from build123d import *

# Parameters (mm, degrees)
SKETCH_1_R          = 5
EXTRUDE_4_DEPTH     = 10
SKETCH_4_R          = 4
EXTRUDE_5_DEPTH     = 10
EXTRUDE_START       = 10
SKETCH_5_R          = 4
EXTRUDE_6_DEPTH     = 10
EXTRUDE_START_2     = -3
SKETCH_6_W          = 4.7
SKETCH_6_H          = 4.7
EXTRUDE_7_DEPTH     = 3
CUT_EXTRUDE_START   = -5
CUT_EXTRUDE_1_DEPTH = 5
SKETCH_8_R          = 1.5
CUT_EXTRUDE_2_DEPTH = 32.98820095


with BuildPart() as part:
    # 草图1 → 凸台-拉伸4 (new body)
    with BuildSketch(Plane(origin=(0, 0, 0), x_dir=(1, 0, 0), z_dir=(0, 1, 0))):
        with Locations(Location((0, 0, 0), (0, 0, 270))):
            Circle(SKETCH_1_R)
    extrude(amount=EXTRUDE_4_DEPTH)

    # 草图4 → 凸台-拉伸5 (add)
    with BuildSketch(Plane(origin=(0, 10, 0), x_dir=(1, 0, 0), z_dir=(0, 1, 0))):
        with Locations(Location((0, 0, 0), (0, 0, 270))):
            Circle(SKETCH_4_R)
    extrude(amount=EXTRUDE_5_DEPTH)

    # 草图5 → 凸台-拉伸6 (add)
    with BuildSketch(Plane.XZ.offset(EXTRUDE_START)):
        with Locations(Location((0, 0, 0), (0, 0, 90))):
            Circle(SKETCH_5_R)
    extrude(amount=-EXTRUDE_6_DEPTH)

    # 草图6 → 凸台-拉伸7 (add)
    with BuildSketch(Plane(origin=(0, 20, 0), x_dir=(1, 0, 0), z_dir=(0, 1, 0)).offset(EXTRUDE_START_2)):
        with BuildLine():
            Line((-7.85, 2.35), (-7.85, -2.35))
            Line((-7.85, -2.35), (-3.236896662, -2.35))
            ThreePointArc((-3.236896662, -2.35), (-4, 0), (-3.236896662, 2.35))
            Line((-3.236896662, 2.35), (-7.85, 2.35))
        make_face()
        with BuildLine():
            Line((-2.35, 7.85), (-2.35, 3.236896662))
            ThreePointArc((-2.35, 3.236896662), (0, 4), (2.35, 3.236896662))
            Line((2.35, 3.236896662), (2.35, 7.85))
            Line((2.35, 7.85), (-2.35, 7.85))
        make_face()
        with BuildLine():
            ThreePointArc((4, 0), (3.804443892, -1.235397376), (3.236896662, -2.35))
            Line((3.236896662, -2.35), (7.85, -2.35))
            Line((7.85, -2.35), (7.85, 2.35))
            Line((7.85, 2.35), (3.236896662, 2.35))
            ThreePointArc((3.236896662, 2.35), (3.804443892, 1.235397376), (4, 0))
        make_face()
        with BuildLine():
            ThreePointArc((2.35, -3.236896662), (0, -4), (-2.35, -3.236896662))
            Line((-2.35, -3.236896662), (-2.35, -7.85))
            Line((-2.35, -7.85), (2.35, -7.85))
            Line((2.35, -7.85), (2.35, -3.236896662))
        make_face()
        with BuildLine():
            Line((2.35, -2.35), (-2.35, -2.35))
            Line((-2.35, -2.35), (-2.35, -3.236896662))
            ThreePointArc((-2.35, -3.236896662), (0, -4), (2.35, -3.236896662))
            Line((2.35, -3.236896662), (2.35, -2.35))
        make_face()
        with BuildLine():
            Line((2.35, 2.35), (2.35, -2.35))
            Line((2.35, -2.35), (3.236896662, -2.35))
            ThreePointArc((3.236896662, -2.35), (3.804443892, -1.235397376), (4, 0))
            ThreePointArc((4, 0), (3.804443892, 1.235397376), (3.236896662, 2.35))
            Line((3.236896662, 2.35), (2.35, 2.35))
        make_face()
        with BuildLine():
            Line((-2.35, 3.236896662), (-2.35, 2.35))
            Line((-2.35, 2.35), (2.35, 2.35))
            Line((2.35, 2.35), (2.35, 3.236896662))
            ThreePointArc((2.35, 3.236896662), (0, 4), (-2.35, 3.236896662))
        make_face()
        with BuildLine():
            ThreePointArc((-3.236896662, 2.35), (-4, 0), (-3.236896662, -2.35))
            Line((-3.236896662, -2.35), (-2.35, -2.35))
            Line((-2.35, -2.35), (-2.35, 2.35))
            Line((-2.35, 2.35), (-3.236896662, 2.35))
        make_face()
        Rectangle(SKETCH_6_W, SKETCH_6_H)
    extrude(amount=EXTRUDE_7_DEPTH)

    # 草图7 → 切除-拉伸1 (cut)
    with BuildSketch(Plane(origin=(0, 20, 0), x_dir=(1, 0, 0), z_dir=(0, 1, 0)).offset(CUT_EXTRUDE_START)):
        with BuildLine():
            Line((-2.35, -2.35), (-3.236896662, -2.35))
            ThreePointArc((-3.236896662, -2.35), (-2.828427125, -2.828427125), (-2.35, -3.236896662))
            Line((-2.35, -3.236896662), (-2.35, -2.35))
        make_face()
        with BuildLine():
            Line((3.236896662, -2.35), (2.35, -2.35))
            Line((2.35, -2.35), (2.35, -3.236896662))
            ThreePointArc((2.35, -3.236896662), (2.828427125, -2.828427125), (3.236896662, -2.35))
        make_face()
        with BuildLine():
            Line((2.35, 3.236896662), (2.35, 2.35))
            Line((2.35, 2.35), (3.236896662, 2.35))
            ThreePointArc((3.236896662, 2.35), (2.828427125, 2.828427125), (2.35, 3.236896662))
        make_face()
        with BuildLine():
            ThreePointArc((-2.35, 3.236896662), (-2.828427125, 2.828427125), (-3.236896662, 2.35))
            Line((-3.236896662, 2.35), (-2.35, 2.35))
            Line((-2.35, 2.35), (-2.35, 3.236896662))
        make_face()
    extrude(amount=CUT_EXTRUDE_1_DEPTH, mode=Mode.SUBTRACT)

    # 草图8 → 切除-拉伸2 (cut, through all)
    with BuildSketch(Plane(origin=(0, 20, 0), x_dir=(1, 0, 0), z_dir=(0, 1, 0))):
        with Locations(Location((0, 0, 0), (0, 0, 270))):
            Circle(SKETCH_8_R)
    extrude(amount=-CUT_EXTRUDE_2_DEPTH, mode=Mode.SUBTRACT)


solid = part.part
The model under review builds one solid part; all positions refer to its coordinate system, in mm. A direction names the side the tool comes from. Round coordinates to 2 decimals unless told otherwise and drop trailing zeros. Order: outer loops, then holes, each group sorted by start corner. A loop starts at its lowest first (then second) coordinate and runs counter-clockwise, first axis right, second up. Notation, with made-up numbers: (55, 9) -> (89, 9) arc R14 ccw to (89, 31) -> close; hole circle Ø1 at (-34, -19). An arc over 180 degrees is marked (long way). Use CSV: the item, a comma, the result in double quotes. Start each with the question number.
(1) Tool access review of faces 5 (the face through (4, 18, -2.35)), 6 (the face through (2.35, 18, 4)), 7 (the face through (-5, 19, 2.35)), 8 (the face through (-4, 18, -2.35)): name each direction out of +Z, -Z, +X, -X, +Y, -Y from which nothing blocks a thin tool from reaching the whole face with its end or side.
(2) Insertion check: pin 1 (4 mm diameter, centred on y = 17, z = 6, fed in from +X); pin 2 (1 mm diameter, centred on x = -4.5, y = 1.5, fed in from +Z); pin 3 (4 mm diameter, centred on x = -4.5, y = 16.5, fed in from -Z). Each pin has a flat end and moves straight along its axis. Give the tip position at first contact, or say it passes through.
(3) Wall thickness on probe 1 along X at (y, z) = (-1.25, 0); probe 2 along X at (y, z) = (0.5, 0); probe 3 along Y at (x, z) = (5.5, -2.25): over which ranges is each line inside the solid? List them lowest first. Write a range as from..to.
(4) Consider section B-B on z = 0. Write out the cut boundary in (x, y).
(5) Consider section C-C on y = 16.25. Write out the cut boundary in (x, z), and give its area (3 significant figures).
(6) Mouldability with a two-part tool opening along Y and no side actions: class faces 1 (the face through (0, 17, -6)), 2 (the face through (0, 18, -7.85)), 3 (the face through (-2.7, 15, -2.7)), 4 (the face through (0, 17, 6)) as pulls with the +Y half, pulls with the -Y half, needs draft (parallel to the pull), parting line crosses it, or undercut.
(7) Consider section D-D on z = -2.75. Write out the cut boundary in (x, y), and give its area (3 significant figures).
(8) Consider section A-A on x = 0. Write out the cut boundary in (y, z).
Responses:
1,face 5,"-Z, +X, +Y"
1,face 6,"+Z, +X, +Y"
1,face 7,"+Z, -X, +Y"
1,face 8,"-Z, -X, +Y"
2,pin 1,"x = 2.35"
2,pin 2,"z = 3"
2,pin 3,"z = -2.43"
3,probe 1,"-4..-1.5, 1.5..4"
3,probe 2,"-5..-1.5, 1.5..5"
3,probe 3,"17..20"
4,outline,"(-7.85, 17) -> (-4, 17) -> (-4, 10) -> (-5, 10) -> (-5, 0) -> (-4, 0) -> (-4, -10) -> (-1.5, -10) -> (-1.5, 20) -> (-7.85, 20) -> close; (1.5, -10) -> (4, -10) -> (4, 0) -> (5, 0) -> (5, 10) -> (4, 10) -> (4, 17) -> (7.85, 17) -> (7.85, 20) -> (1.5, 20) -> close"
5,outline,"(-3.24, -2.35) -> (-2.35, -2.35) -> (-2.35, -3.24) arc R4 ccw to (2.35, -3.24) -> (2.35, -2.35) -> (3.24, -2.35) arc R4 ccw to (3.24, 2.35) -> (2.35, 2.35) -> (2.35, 3.24) arc R4 ccw to (-2.35, 3.24) -> (-2.35, 2.35) -> (-3.24, 2.35) arc R4 ccw to start; hole circle Ø3 at (0, 0)"
5,area,"41.5 mm²"
6,face 1,"undercut"
6,face 2,"needs draft"
6,face 3,"pulls with the +Y half"
6,face 4,"undercut"
7,outline,"(-4.18, 0) -> (-2.9, 0) -> (-2.9, -10) -> (2.9, -10) -> (2.9, 0) -> (4.18, 0) -> (4.18, 10) -> (2.9, 10) -> (2.9, 15) -> (2.35, 15) -> (2.35, 20) -> (-2.35, 20) -> (-2.35, 15) -> (-2.9, 15) -> (-2.9, 10) -> (-4.18, 10) -> close"
7,area,"194 mm²"
8,outline,"(-10, -4) -> (0, -4) -> (0, -5) -> (10, -5) -> (10, -4) -> (17, -4) -> (17, -7.85) -> (20, -7.85) -> (20, -1.5) -> (-10, -1.5) -> close; (-10, 1.5) -> (20, 1.5) -> (20, 7.85) -> (17, 7.85) -> (17, 4) -> (10, 4) -> (10, 5) -> (0, 5) -> (0, 4) -> (-10, 4) -> close"
